from build123d import *

# Parameters (mm, degrees)
SKETCH_1_R          = 2.5
EXTRUDE_1_DEPTH     = 371
CUT_EXTRUDE_1_DEPTH = 372.673243589
SKETCH_3_W          = 49.042761982
SKETCH_3_H          = 45.736729066
CUT_EXTRUDE_2_DEPTH = 240


with BuildPart() as part:
    # 草图1 → 凸台-拉伸1 (new body)
    with BuildSketch(Plane.XY):
        with BuildLine():
            Line((-8.2, -3.1), (-10, -3.1))
            Line((-10, -3.1), (-10, -8.5))
            ThreePointArc((-10, -8.5), (-9.560660172, -9.560660172), (-8.5, -10))
            Line((-8.5, -10), (-3.1, -10))
            Line((-3.1, -10), (-3.1, -8.2))
            Line((-3.1, -8.2), (-5.5, -8.2))
            Line((-5.5, -8.2), (-5.5, -6.397050155))
            Line((-5.5, -6.397050155), (-2.202949845, -3.1))
            Line((-2.202949845, -3.1), (2.202949845, -3.1))
            Line((2.202949845, -3.1), (5.5, -6.397050155))
            Line((5.5, -6.397050155), (5.5, -8.2))
            Line((5.5, -8.2), (3.1, -8.2))
            Line((3.1, -8.2), (3.1, -10))
            Line((3.1, -10), (8.5, -10))
            ThreePointArc((8.5, -10), (9.560660172, -9.560660172), (10, -8.5))
            Line((10, -8.5), (10, -3.1))
            Line((10, -3.1), (8.2, -3.1))
            Line((8.2, -3.1), (8.2, -5.5))
            Line((8.2, -5.5), (6.397050155, -5.5))
            Line((6.397050155, -5.5), (3.05412702, -2.157076865))
            Line((3.05412702, -2.157076865), (3.05412702, 2.157076865))
            Line((3.05412702, 2.157076865), (6.397050155, 5.5))
            Line((6.397050155, 5.5), (8.2, 5.5))
            Line((8.2, 5.5), (8.2, 3.1))
            Line((8.2, 3.1), (10, 3.1))
            Line((10, 3.1), (10, 8.5))
            ThreePointArc((10, 8.5), (9.560660172, 9.560660172), (8.5, 10))
            Line((8.5, 10), (3.1, 10))
            Line((3.1, 10), (3.1, 8.2))
            Line((3.1, 8.2), (5.5, 8.2))
            Line((5.5, 8.2), (5.5, 6.397050155))
            Line((5.5, 6.397050155), (2.202949845, 3.1))
            Line((2.202949845, 3.1), (-2.202949845, 3.1))
            Line((-2.202949845, 3.1), (-5.5, 6.397050155))
            Line((-5.5, 6.397050155), (-5.5, 8.2))
            Line((-5.5, 8.2), (-3.1, 8.2))
            Line((-3.1, 8.2), (-3.1, 10))
            Line((-3.1, 10), (-8.5, 10))
            ThreePointArc((-8.5, 10), (-9.560660172, 9.560660172), (-10, 8.5))
            Line((-10, 8.5), (-10, 3.1))
            Line((-10, 3.1), (-8.2, 3.1))
            Line((-8.2, 3.1), (-8.2, 5.5))
            Line((-8.2, 5.5), (-6.397050155, 5.5))
            Line((-6.397050155, 5.5), (-3.05412702, 2.157076865))
            Line((-3.05412702, 2.157076865), (-3.05412702, -2.157076865))
            Line((-3.05412702, -2.157076865), (-6.397050155, -5.5))
            Line((-6.397050155, -5.5), (-8.2, -5.5))
            Line((-8.2, -5.5), (-8.2, -3.1))
        make_face()
        Circle(SKETCH_1_R, mode=Mode.SUBTRACT)
    extrude(amount=EXTRUDE_1_DEPTH)

    # 草图2 → 切除-拉伸1 (cut, through all)
    with BuildSketch(Plane(origin=(0, 10, 0), x_dir=(1, 0, 0), z_dir=(0, 1, 0))):
        Polygon((10, 0), (10, -20), (-10, 0), align=None)
    extrude(amount=-CUT_EXTRUDE_1_DEPTH, mode=Mode.SUBTRACT)

    # 草图3 → 切除-拉伸2 (cut)
    with BuildSketch(Plane.XY.offset(371)):
        with Locations((9.560660172, -9.560660172)):
            Rectangle(SKETCH_3_W, SKETCH_3_H)
    extrude(amount=-CUT_EXTRUDE_2_DEPTH, mode=Mode.SUBTRACT)


solid = part.part
Build history of the part. All positions in model axes, mm. A direction names the side the tool comes from. Round coordinates to 2 decimals unless told otherwise and drop trailing zeros. Loops run counter-clockwise (first coordinate to the right, second up) from the corner with the lowest first, then second, coordinate; pieces in that order, holes last. Notation, with made-up numbers: (-32.75, 41) -> (8.25, 41) arc R33 ccw to (8.25, 72) -> close; hole circle Ø9 at (-33, 14.25). An arc over 180 degrees is marked (long way). One line per item, written item: value. Start each with the question number.
Q1. Cut at B-B on y = 0. List the corners of the cut face in (x, z).
Q2. Cut at A-A on x = 0. List the corners of the cut face in (y, z), plus the area to 3 significant figures.
Q3. Probe line 1 along Y through (x, z) = (-1.25, 110); line 2 along Y through (x, z) = (-6.5, 54.5); line 3 along X through (y, z) = (0, 86). List the from-to ranges inside material, lowest first.
Q4. Two-plate mould, pull along Y, no slides. Class faces 1 (the face through (10, -6, 75)), 2 (the face through (0, 3.1, 69)), 3 (the face through (-3.828, 4.725, 66.864)): released by +Y, released by -Y, zero draft, split by the parting line, or undercut.
Q5. 3-axis set-ups, long thin cutter, end or side, ignore diameter. For faces 4 (the face through (-4, -8.2, 67)), 5 (the face through (3.054, 0, 71)), 6 (the face through (-2, 2, 131)), 7 (the face through (-3.054, 0, 68)): which of +Z, -Z, +X, -X, +Y, -Y reach the whole face in a straight line?
Q6. Drop flat-ended pins along their axis: pin 1 Ø6 at (x, y) = (4.5, 1) entering from -Z; pin 2 Ø3.5 at (y, z) = (0.5, 99) entering from +X; pin 3 Ø2 at (y, z) = (0.5, 71) entering from -X. Give the stop position or say it passes through.
Computed:
1. outline: (-3.05, 6.95) -> (-2.5, 7.5) -> (-2.5, 131) -> (-3.05, 131) -> close; (2.5, 12.5) -> (3.05, 13.05) -> (3.05, 131) -> (2.5, 131) -> close
2. outline: (-3.1, 10) -> (-2.5, 10) -> (-2.5, 131) -> (-3.1, 131) -> close; (2.5, 10) -> (3.1, 10) -> (3.1, 131) -> (2.5, 131) -> close
2. area: 145 mm²
3. line 1: -3.1 to -2.17, 2.17 to 3.1
3. line 2: -10 to -5.5, 5.5 to 10
3. line 3: -3.05 to -2.5, 2.5 to 3.05
4. face 1: zero draft
4. face 2: released by +Y
4. face 3: undercut
5. face 4: +Z, -Z
5. face 5: +Z, -Z, +X
5. face 6: +Z, +X, -X, +Y, -Y
5. face 7: +Z, -Z, -X
6. pin 1: z = 11.64
6. pin 2: x = 3.15
6. pin 3: x = -3.05
